```python
from build123d import *

# Parameters (mm, degrees)
F1_DEPTH  = 14
F2_R      = 5
F3_R      = 20.5
F4_DEPTH  = 10
F7_DEPTH  = 35.5
F10_DEPTH = 106.1


with BuildPart() as f1:
    # F0 (on Front) → F1 (new body)
    with BuildSketch(Plane.XZ):
        with BuildLine():
            ThreePointArc((45.5, 24.999816), (38.609496, 16.288102), (28, 13))
            Line((28, 13), (-28, 13))
            ThreePointArc((-28, 13), (-38.609496, 16.288102), (-45.5, 24.999816))
            ThreePointArc((-45.5, 24.999816), (-48.595144, 42.322464), (-57.5, 57.5))
            ThreePointArc((-57.5, 57.5), (-72.676021, 34.519669), (-78, 7.5))
            ThreePointArc((-78, 7.5), (-71.995689, -6.995689), (-57.5, -13))
            Line((-57.5, -13), (-28, -13))
            Line((-28, -13), (28, -13))
            Line((28, -13), (57.5, -13))
            ThreePointArc((57.5, -13), (71.995689, -6.995689), (78, 7.5))
            ThreePointArc((78, 7.5), (72.676021, 34.519669), (57.5, 57.5))
            ThreePointArc((57.5, 57.5), (48.595144, 42.322464), (45.5, 24.999816))
        make_face()
    extrude(amount=F1_DEPTH)

    # F2
    f2_edges = [f1.edges().sort_by_distance(p)[0] for p in [
        (57.5, -7, 57.5),
        (-57.5, -7, 57.5),
    ]]
    fillet(f2_edges, radius=F2_R)

    # F3 (on face) → F4 (cut)
    with BuildSketch(Plane.XZ.offset(14)):
        with Locations((57.5, 7.5)):
            Circle(F3_R)
    extrude(amount=-F4_DEPTH, mode=Mode.SUBTRACT)

    # F6 (on offset) → F7 (cut)
    with BuildSketch(Plane.YZ.offset(78.5)):
        Polygon((-16.908804, 57.223689), (-16.908804, 6.107894), (-7.749326, 5.516961), (-2.578652, 57.223689), align=None)
    extrude(amount=-F7_DEPTH, mode=Mode.SUBTRACT)

    # F9 (on offset) → F10 (join)
    with BuildSketch(Plane.YZ.offset(57)):
        Polygon((0, 0), (0, 6.538654), (0, 28.561684), (-1.554986, 28.561684), (-3.524526, 10.537416), (-3.524526, 0), align=None)
    extrude(amount=-F10_DEPTH)


solid = f1.part
```
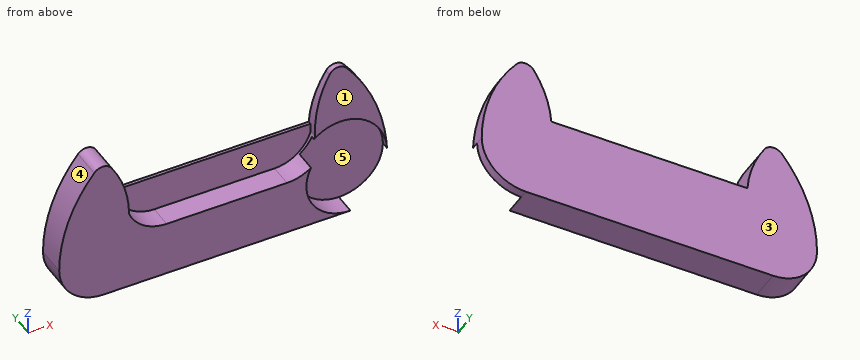
For this review, take the finished solid that the model builds, in its own axes (mm). Face numbers are marked on the shaded views. A direction names the side the tool comes from. Give positions to 0.01 mm unless a question says otherwise; leave off trailing zeros. Write each loop counter-clockwise with the first axis right and the second up, starting at its lowest first coordinate (ties: lowest second). Pieces come first, ordered by that corner, then holes.
Item 1: Take a section at B-B (x = -4.5). Give the boundary of the cut face in (y, z), and give its area (3 significant figures).
Item 2: Insertion check: P1, Ø5, axis at y = -8, z = 26, coming from the -X side; P2, Ø1.7, axis at x = -22.5, y = -1, coming from the +Z side; P3, Ø3, axis at y = -3, z = 19, coming from the +X side. Each pin has a flat end and moves straight along its axis. Give the tip position at first contact, or say it passes through.
Item 3: Take a section at A-A (z = 42.5). Give the boundary of the cut face in (x, y).
Item 4: Take a section at D-D (x = 42). Give the boundary of the cut face in (y, z), and give its area (3 significant figures).
Item 5: Take a section at C-C (z = 33). Give the boundary of the cut face in (x, y).
Item 6: Machinability: for the marked faces 1, 2, 3, 4 and 5, which of the approach directions +Z, -Z, +X, -X, +Y, -Y give a long, thin tool a straight path to every point of the face, cutting with its end or side? Answer none if there is none.
Item 7: Wall thickness on probe 1 along Z at (x, y) = (-27.5, -9.75); probe 2 along Y at (x, z) = (50, -9); probe 3 along Z at (x, y) = (-6, -1.25): over which ranges is each line inside the solid? List them lowest first.
Established:
1. outline: (-14, -13) - (0, -13) - (0, 28.56) - (-1.55, 28.56) - (-3.26, 13) - (-14, 13) - close
1. area: 401 mm2
2. P1: stops at x = -76.18
2. P2: stops at z = 28.56
2. P3: stops at x = 77.29
3. outline: (-68.81, -14) - (-48.66, -14) - (-48.66, 0) - (-68.81, 0) - close; (48.66, -4.05) - (68.81, -4.05) - (68.81, 0) - (48.66, 0) - close
4. outline: (-14, -13) - (0, -13) - (0, 28.56) - (-1.55, 28.56) - (-2.57, 19.27) - (-4, 19.27) - (-4, -5.92) - (-14, -5.92) - close
4. area: 219 mm2
5. outline: (-73.28, -14) - (-46.14, -14) - (-46.14, 0) - (-73.28, 0) - close; (46.14, -5) - (73.28, -5) - (73.28, 0) - (46.14, 0) - close
6. face 1: +Z, +X, -Y
6. face 2: +Z, -Y
6. face 3: +Z, -Z, +X, -X, +Y
6. face 4: +Z, -X, +Y, -Y
6. face 5: -Y
7. probe 1: z = -13 to 13
7. probe 2: y = -4 to 0
7. probe 3: z = -13 to 28.56
